```python
from build123d import *

# Parameters (mm, degrees)
SALIENTE_EXTRUIR3_DEPTH = 6.35
CROQUIS5_W              = 2.54
CROQUIS5_H              = 196.85
CORTAR_EXTRUIR1_DEPTH   = 6.35


with BuildPart() as part:
    # Croquis2 → Saliente-Extruir3 (new body)
    with BuildSketch(Plane.XY):
        with BuildLine():
            Line((0, 0), (6.35, 0))
            Line((6.35, 0), (6.35, -6.35))
            Line((6.35, -6.35), (82.55, -6.35))
            Line((82.55, -6.35), (82.55, 0))
            Line((82.55, 0), (88.9, 0))
            Line((88.9, 0), (88.9, 50.8))
            ThreePointArc((88.9, 50.8), (83.320384182, 64.270384182), (69.85, 69.85))
            Line((69.85, 69.85), (63.5, 69.85))
            ThreePointArc((63.5, 69.85), (50.029615818, 75.429615818), (44.45, 88.9))
            Line((44.45, 88.9), (44.45, 190.5))
            ThreePointArc((44.45, 190.5), (38.870384182, 203.970384182), (25.4, 209.55))
            Line((25.4, 209.55), (0, 209.55))
            Line((0, 209.55), (0, 203.2))
            Line((0, 203.2), (-6.35, 203.2))
            Line((-6.35, 203.2), (-6.35, 6.35))
            Line((-6.35, 6.35), (0, 6.35))
            Line((0, 6.35), (0, 0))
        make_face()
    extrude(amount=SALIENTE_EXTRUIR3_DEPTH)

    # Croquis5 → Cortar-Extruir1 (cut)
    with BuildSketch(Plane.ZY.offset(6.35)):
        with Locations((1.27, 104.775)):
            Rectangle(CROQUIS5_W, CROQUIS5_H)
    extrude(amount=-CORTAR_EXTRUIR1_DEPTH, mode=Mode.SUBTRACT)


solid = part.part
```
Here's how the part is built. I have some questions about the finished solid (model axes, mm). A direction names the side the tool comes from. Round coordinates to 2 decimals unless told otherwise and drop trailing zeros. Order: outer loops, then holes, each group sorted by start corner. A loop starts at its lowest first (then second) coordinate and runs counter-clockwise, first axis right, second up. Notation, with made-up numbers: M 86,88.5 L 138,88.5 A34 cw 138,121.5 Z; hole C -0.75,61 d4. An arc over 180 degrees is marked long. Answer as CSV lines item,"result".
Item 1: Imagine slicing it at B-B on z = 4.25. List the corners of the cut face in (x, y) for me, and give its area (3 significant figures).
From the geometry:
outline,"M -6.35,6.35 L 0,6.35 L 0,0 L 6.35,0 L 6.35,-6.35 L 82.55,-6.35 L 82.55,0 L 88.9,0 L 88.9,50.8 A19.05 ccw 69.85,69.85 L 63.5,69.85 A19.05 cw 44.45,88.9 L 44.45,190.5 A19.05 ccw 25.4,209.55 L 0,209.55 L 0,203.2 L -6.35,203.2 Z"
area,"14,100 mm2"
Item 2: For pin 1 (1.9 mm diameter, centred on x = 2.5, z = 3, fed in from -Y); pin 2 (1.1 mm diameter, centred on x = -3, z = 3.5, fed in from -Y); pin 3 (2 mm diameter, centred on y = 104.5, z = 1.5, fed in from +X); pin 4 (1.5 mm diameter, centred on x = 6, y = 22.5, fed in from -Z), each with a flat end and sliding along its axis, tell me the tip position at first contact or that it passes through.
From the geometry:
pin 1,"y = 0"
pin 2,"y = 6.35"
pin 3,"x = 44.45"
pin 4,"z = 0"
Item 3: Please list where these lines run through material, in increasing order: L1, parallel to X at y = 93, z = 4; L2, parallel to X at y = 51, z = 0.5; L3, parallel to Z at x = -1, y = 101. Write a range as [from, to].
From the geometry:
L1,"[-6.35, 44.45]"
L2,"[0, 88.9]"
L3,"[2.54, 6.35]"
Item 4: Which directions (+Z, -Z, +X, -X, +Y, -Y) give clear straight access to the entire face, cutting with the end or side of a thin tool? Please do faces 1 (the flat face through (6.35, -3, 3)), 2 (the flat face through (44.45, 139, 3)), 3 (the flat face through (-3, 203.2, 4)), 4 (the flat face through (82.55, -3, 3)).
From the geometry:
face 1,"+Z, -Z, -X, -Y"
face 2,"+Z, -Z, +X, +Y"
face 3,"+Z, -Z, -X, +Y"
face 4,"+Z, -Z, +X, -Y"
Item 5: Imagine slicing it at A-A on y = 175.5. List the corners of the cut face in (x, z) for me, and give its area (3 significant figures).
From the geometry:
outline,"M -6.35,2.54 L 0,2.54 L 0,0 L 44.45,0 L 44.45,6.35 L -6.35,6.35 Z"
area,"306 mm2"
Item 6: Imagine slicing it at D-D on x = 37. List the corners of the cut face in (y, z) for me, and give its area (3 significant figures).
From the geometry:
outline,"M -6.35,0 L 205.61,0 L 205.61,6.35 L -6.35,6.35 Z"
area,"1,350 mm2"
Item 7: Imagine slicing it at C-C on y = 39. List the corners of the cut face in (x, z) for me, and give its area (3 significant figures).
From the geometry:
outline,"M -6.35,2.54 L 0,2.54 L 0,0 L 88.9,0 L 88.9,6.35 L -6.35,6.35 Z"
area,"589 mm2"
